```python
from build123d import *

# Parameters (mm, degrees)
F0_W     = 609.6
F0_H     = 457.2
F1_DEPTH = 914.4
F2_W     = 603.25
F2_H     = 908.05
F3_DEPTH = 452.755
F4_W     = 603.25
F4_H     = 73.025
F4_H_2   = 225.425
F4_H_3   = 220.98
F5_DEPTH = 454.025
F7_DEPTH = 25.4


with BuildPart() as f1:
    # F0 (on Top) → F1 (new body)
    with BuildSketch(Plane.XY):
        Rectangle(F0_W, F0_H)
    extrude(amount=F1_DEPTH)

    # F2 (on face) → F3 (cut)
    with BuildSketch(Plane.XZ.offset(228.6)):
        with Locations((0, 457.2)):
            Rectangle(F2_W, F2_H)
    extrude(amount=-F3_DEPTH, mode=Mode.SUBTRACT)

    # F4 (on face) → F5 (join)
    with BuildSketch(Plane.XZ.offset(-224.155)):
        with Locations((0, 874.7125)):
            Rectangle(F4_W, F4_H)
        with Locations((0, 798.5125)):
            Rectangle(F4_W, F4_H)
        with Locations((0, 722.3125)):
            Rectangle(F4_W, F4_H)
        with Locations((0, 569.9125)):
            Rectangle(F4_W, F4_H_2)
        with Locations((0, 341.3125)):
            Rectangle(F4_W, F4_H_2)
        with Locations((0, 114.935)):
            Rectangle(F4_W, F4_H_3)
    extrude(amount=F5_DEPTH)

    # F6 (on face) → F7 (cut)
    with BuildSketch(Plane.XZ.offset(229.87)):
        with BuildLine():
            Line((76.2, 906.4625), (0, 906.4625))
            Line((0, 906.4625), (0, 842.9625))
            Line((0, 842.9625), (76.2, 842.9625))
            ThreePointArc((76.2, 842.9625), (107.95, 874.7125), (76.2, 906.4625))
        make_face()
        with BuildLine():
            Line((0, 842.9625), (0, 906.4625))
            Line((0, 906.4625), (-76.2, 906.4625))
            ThreePointArc((-76.2, 906.4625), (-107.95, 874.7125), (-76.2, 842.9625))
            Line((-76.2, 842.9625), (0, 842.9625))
        make_face()
        with BuildLine():
            Line((76.2, 220.6498), (0, 220.6498))
            Line((0, 220.6498), (0, 157.1498))
            Line((0, 157.1498), (76.2, 157.1498))
            ThreePointArc((76.2, 157.1498), (107.95, 188.8998), (76.2, 220.6498))
        make_face()
        with BuildLine():
            Line((0, 157.1498), (0, 220.6498))
            Line((0, 220.6498), (-76.2, 220.6498))
            ThreePointArc((-76.2, 220.6498), (-107.95, 188.8998), (-76.2, 157.1498))
            Line((-76.2, 157.1498), (0, 157.1498))
        make_face()
        with BuildLine():
            Line((76.2, 449.2498), (0, 449.2498))
            Line((0, 449.2498), (0, 385.7498))
            Line((0, 385.7498), (76.2, 385.7498))
            ThreePointArc((76.2, 385.7498), (107.95, 417.4998), (76.2, 449.2498))
        make_face()
        with BuildLine():
            Line((0, 385.7498), (0, 449.2498))
            Line((0, 449.2498), (-76.2, 449.2498))
            ThreePointArc((-76.2, 449.2498), (-107.95, 417.4998), (-76.2, 385.7498))
            Line((-76.2, 385.7498), (0, 385.7498))
        make_face()
        with BuildLine():
            Line((76.2, 677.8498), (0, 677.8498))
            Line((0, 677.8498), (0, 614.3498))
            Line((0, 614.3498), (76.2, 614.3498))
            ThreePointArc((76.2, 614.3498), (107.95, 646.0998), (76.2, 677.8498))
        make_face()
        with BuildLine():
            Line((0, 614.3498), (0, 677.8498))
            Line((0, 677.8498), (-76.2, 677.8498))
            ThreePointArc((-76.2, 677.8498), (-107.95, 646.0998), (-76.2, 614.3498))
            Line((-76.2, 614.3498), (0, 614.3498))
        make_face()
        with BuildLine():
            Line((76.2, 754.0498), (0, 754.0498))
            Line((0, 754.0498), (0, 690.5498))
            Line((0, 690.5498), (76.2, 690.5498))
            ThreePointArc((76.2, 690.5498), (107.95, 722.2998), (76.2, 754.0498))
        make_face()
        with BuildLine():
            Line((0, 690.5498), (0, 754.0498))
            Line((0, 754.0498), (-76.2, 754.0498))
            ThreePointArc((-76.2, 754.0498), (-107.95, 722.2998), (-76.2, 690.5498))
            Line((-76.2, 690.5498), (0, 690.5498))
        make_face()
        with BuildLine():
            Line((76.2, 830.2498), (0, 830.2498))
            Line((0, 830.2498), (0, 766.7498))
            Line((0, 766.7498), (76.2, 766.7498))
            ThreePointArc((76.2, 766.7498), (107.95, 798.4998), (76.2, 830.2498))
        make_face()
        with BuildLine():
            Line((0, 766.7498), (0, 830.2498))
            Line((0, 830.2498), (-76.2, 830.2498))
            ThreePointArc((-76.2, 830.2498), (-107.95, 798.4998), (-76.2, 766.7498))
            Line((-76.2, 766.7498), (0, 766.7498))
        make_face()
    extrude(amount=-F7_DEPTH, mode=Mode.SUBTRACT)


solid = f1.part
```
Read the model definition and answer for the solid it produces. Units are mm, in the model's axes. A direction names the side the tool comes from. Give positions to 0.01 mm unless a question says otherwise; leave off trailing zeros. Write each loop counter-clockwise with the first axis right and the second up, starting at its lowest first coordinate (ties: lowest second). Pieces come first, ordered by that corner, then holes. Notation, with made-up numbers: M -17.5,82 L 36.5,82 A11 cw 36.5,92 Z; hole C -24,32 d9. An arc over 180 degrees is marked long. Put each result on its own line as item: value. Start each with the question number.
1. For a pull along Z with two mould halves and no side action, classify faces 3 (the flat face through (-2, -204.47, 723)), 4 (the flat face through (-4, 3, 0)), 5 (the flat face through (304.8, -3, 451)) as released by +Z, released by -Z, zero draft, split by the parting line, or undercut.
2. The part is cut by section A-A, the plane y = 31. Give the vertices of the cut face in (x, z) (3 decimals).
3. Consider line 1 along Y through (x, z) = (17, 807). Determine where the line is inside the solid, lowest interval first.
4. This flat-tipped pin is pushed along its axis until it touches: pin 1 Ø1 at (y, z) = (-229.5, 163.5) entering from +X (3 decimals). Where does it stop, or does it pass through?
5. The part is cut by section B-B, the plane z = 783.5. Give the vertices of the cut face in (x, y) (3 decimals).
6. Which of the six approach directions +Z, -Z, +X, -X, +Y, -Y give full straight-line access (tool end or side, diameter ignored) to faces 1 (the flat face through (-4, 3, 914.4)), 2 (the flat face through (-1, -217, 842.962))?
Final values:
1. face 3: undercut
1. face 4: released by -Z
1. face 5: zero draft
2. outline: M -304.8,0 L 304.8,0 L 304.8,914.4 L -304.8,914.4 Z; hole M -301.625,3.175 L 301.625,3.175 L 301.625,4.445 L -301.625,4.445 Z; hole M -301.625,225.425 L 301.625,225.425 L 301.625,228.6 L -301.625,228.6 Z; hole M -301.625,454.025 L 301.625,454.025 L 301.625,457.2 L -301.625,457.2 Z; hole M -301.625,682.625 L 301.625,682.625 L 301.625,685.8 L -301.625,685.8 Z; hole M -301.625,758.825 L 301.625,758.825 L 301.625,762 L -301.625,762 Z; hole M -301.625,835.025 L 301.625,835.025 L 301.625,838.2 L -301.625,838.2 Z
3. line 1: y = -204.47 to 228.6
4. pin 1: stops at x = 301.625
5. outline: M -304.8,-228.6 L -301.625,-228.6 L -301.625,-229.87 L -104.183,-229.87 L -104.183,-204.47 L 104.183,-204.47 L 104.183,-229.87 L 301.625,-229.87 L 301.625,-228.6 L 304.8,-228.6 L 304.8,228.6 L -304.8,228.6 Z
6. face 1: +Z, +X, -X, +Y, -Y
6. face 2: -Y
